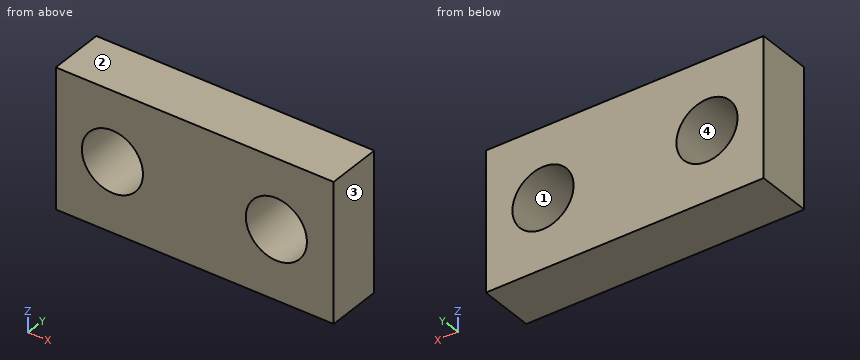
Autodesk Inventor part; units mm, degrees
ref_plane "YZ Plane" through (0, 0, 0) normal (1, 0, 0) x (0, 1, 0)
ref_plane "XZ Plane" through (0, 0, 0) normal (0, 1, 0) x (-1, 0, 0)
ref_plane "XY Plane" through (0, 0, 0) normal (0, 0, 1) x (1, 0, 0)
sketch "Spacer 2D" plane through (0, 0, 0) normal (0, 1, 0) x (-1, 0, 0)
  line L0 (0, -6.35) -> (26.162, -6.35) construction
  line L1 (13.0671, 0) -> (13.0671, -12.7) construction
  line L2 (25.7671, -12.7) -> (0.3671, -12.7)
  line L3 (0.3671, -12.7) -> (0.3671, 0)
  line L4 (0.3671, 0) -> (25.7671, 0)
  line L5 (25.7671, 0) -> (25.7671, -12.7)
  line L6 (25.7671, -12.7) -> (0.3671, 0) construction
  line L7 (0.3671, -12.7) -> (25.7671, 0) construction
  line L8 (13.081, -12.7) -> (13.081, 0) construction
  line L9 (25.7949, -12.7) -> (25.7949, 0) construction
  line L10 (17.78, -6.35) -> (24.8285, -6.35) construction
  line L11 (17.78, -6.35) -> (23.368, -6.35) construction
  circle A0 centre (20.574, -6.35) radius 2.794
  circle A1 centre (5.588, -6.35) radius 2.794
  line L12 (8.382, -6.35) -> (17.78, -6.35) construction
  line L13 (0.3949, 0) -> (0.3949, -12.7) construction
  line L14 (0.381, -12.7) -> (25.781, -12.7) construction
  line L15 (25.781, -12.7) -> (25.781, 0) construction
  line L16 (25.781, 0) -> (0.381, 0) construction
  line L17 (0.381, 0) -> (0.381, -12.7) construction
  line L18 (0.381, -12.7) -> (25.781, 0) construction
  line L19 (25.781, -12.7) -> (0.381, 0) construction
  point P0 (0, 0)
  point P1 (13.0671, -6.35)
  point P2 (13.081, -6.35)
  dimension "d17" = 25.4
  dimension "d18" = 12.7
  dimension "d31" = 5.588
  dimension "d32" = 9.398
  dimension "d33" = 8.001
  dimension "d34" = 8.001
  dimension "d35" = 2.4269
  dimension "d36" = 2.4269
extrude "Spacer Body" add sketch "Spacer 2D" along normal blind 5.08 contours L2 L3 L4 L5 | A0 | A1
sketch "Spacer Circles" plane through (0, 5.08, 0) normal (0, 1, 0) x (1, 0, 0)
  line L0 (-13.0949, 0) -> (-13.0949, 12.7) construction
  line L1 (-0.3671, 0) -> (-0.3671, 12.7) construction
  circle A0 centre (-5.6019, 6.35) radius 2.794
  circle A1 centre (-20.5879, 6.35) radius 2.794
  line L2 (-17.7939, 6.35) -> (-8.3959, 6.35) construction
  line L3 (-25.7671, 12.7) -> (-25.7671, 0) construction
  line L4 (-25.7949, 0) -> (-0.3949, 0) construction
  line L5 (-0.3949, 0) -> (-0.3949, 12.7) construction
  line L6 (-0.3949, 12.7) -> (-25.7949, 12.7) construction
  line L7 (-25.7949, 12.7) -> (-25.7949, 0) construction
  line L8 (-25.7949, 0) -> (-0.3949, 12.7) construction
  line L9 (-0.3949, 0) -> (-25.7949, 12.7) construction
  point P0 (-13.0949, 6.35)
  dimension "d26" = 9.398
  dimension "d29" = 8.001
  dimension "d30" = 8.001
extrude "Spacer Holes" cut sketch "Spacer Circles" against normal blind 10.16
equation "\"d36\" = d35"
properties part number "Rectangular Top Washer v1.2"
Could you check a few things on this model? Use its own coordinates, in mm. Face numbers are marked on the shaded views. Give positions to 0.01 mm unless a question says otherwise; leave off trailing zeros. Order: outer loops, then holes, each group sorted by start corner. A loop starts at its lowest first (then second) coordinate and runs counter-clockwise, first axis right, second up.
Item 1: I'm going to push flat-ended pins straight in: pin 1 (1 mm diameter, centred on x = -9, y = 4.5, fed in from +Z); pin 2 (4.5 mm diameter, centred on x = -20.59, z = -6.35, fed in from -Y). Where does each tip first touch, or does it pass through?
Item 2: If we section it at C-C, the plane x = -21: Write out the boundary of the cut face in (y, z), plus the area to 3 significant figures.
Item 3: If we mould it in two halves opening along Z, with no side actions, what happens to the marked faces 1, 2, 3 and 4? For each: pulls with the +Z half, pulls with the -Z half, needs draft (parallel to the pull), parting line crosses it, or undercut.
Item 4: If we section it at D-D, the plane z = -7.75: Write out the boundary of the cut face in (x, y).
Item 5: I need wall thicknesses on line 1 (X direction, y = 2.35, z = -6.35); line 2 (X direction, y = 4.05, z = -7.5); line 3 (Z direction, x = -7.25, y = 0.9). Which ranges of each line are inside material? Lowest first, please.
Item 6: If we section it at A-A, the plane z = -6.35: Write out the boundary of the cut face in (x, y).
Item 7: If we section it at B-B, the plane y = 0.7: Write out the boundary of the cut face in (x, z).
Values:
1. pin 1: stops at z = 0
1. pin 2: passes through
2. outline: (0, -12.7) - (5.08, -12.7) - (5.08, -9.11) - (0, -9.11) - close; (0, -3.59) - (5.08, -3.59) - (5.08, 0) - (0, 0) - close
2. area: 36.4 mm2
3. face 1: undercut
3. face 2: pulls with the +Z half
3. face 3: needs draft
3. face 4: undercut
4. outline: (-25.77, 0) - (-23.01, 0) - (-23.01, 5.08) - (-25.77, 5.08) - close; (-18.17, 0) - (-8.02, 0) - (-8.02, 5.08) - (-18.17, 5.08) - close; (-3.18, 0) - (-0.37, 0) - (-0.37, 5.08) - (-3.18, 5.08) - close
5. line 1: x = -25.77 to -23.38, -17.79 to -8.4, -2.81 to -0.37
5. line 2: x = -25.77 to -23.13, -18.04 to -8.15, -3.06 to -0.37
5. line 3: z = -12.7 to -8.61, -4.09 to 0
6. outline: (-25.77, 0) - (-23.38, 0) - (-23.38, 5.08) - (-25.77, 5.08) - close; (-17.79, 0) - (-8.4, 0) - (-8.4, 5.08) - (-17.79, 5.08) - close; (-2.81, 0) - (-0.37, 0) - (-0.37, 5.08) - (-2.81, 5.08) - close
7. outline: (-25.77, -12.7) - (-0.37, -12.7) - (-0.37, 0) - (-25.77, 0) - close; hole circle Ø5.59 at (-20.59, -6.35); hole circle Ø5.59 at (-5.6, -6.35)
